```python
from build123d import *

# Parameters (mm, degrees)
F2_T = -2.54


with BuildPart() as f1:
    # F0 (on Right) → F1 (revolve)
    with BuildSketch(Plane.YZ):
        with BuildLine():
            Line((-101.6, 0), (0, 0))
            Line((0, 0), (0, 635))
            Line((0, 635), (-79.028264, 460.275492))
            ThreePointArc((-79.028264, 460.275492), (-95.892951, 409.140737), (-101.6, 355.6))
            Line((-101.6, 355.6), (-101.6, 0))
        make_face()
    revolve(axis=Axis((0, 0, 317.5), (0, 0, 1)))

    # F2
    f2_openings = [f1.faces().sort_by_distance(p)[0] for p in [
        (0, 0, 0),
    ]]
    offset(amount=F2_T, openings=f2_openings)


solid = f1.part
```
CAD build for the part. Positions are in the model's coordinates, mm. Round coordinates to 2 decimals unless told otherwise and drop trailing zeros. Write each loop counter-clockwise with the first axis right and the second up, starting at its lowest first coordinate (ties: lowest second). Pieces come first, ordered by that corner, then holes. Notation, with made-up numbers: (80, 42) -> (99, 42) arc R20 cw to (99, 63) -> close; hole circle Ø8 at (-6, -30.75). An arc over 180 degrees is marked (long way). Answer in a Markdown table with one row per item. Add a question column.
Item 1: Mould opens along Y. For faces 1 (the face through (-99.184, 22.025, 175.311)), 2 (the face through (30.1, 4, 561.7)), 3 (the face through (98.217, 12.896, 175.311)), 4 (the face through (-97, -22, 0)) say: pulls with the +Y half, pulls with the -Y half, needs draft (parallel to the pull), parting line crosses it, or undercut.
Item 2: Saw through at A-A, the plane z = 195. Write the cut outline in (x, y).
Item 3: Drill centre lines: line 1 (X direction, y = 0, z = 227); line 2 (X direction, y = 20.5, z = 464); line 3 (Y direction, x = 44.5, z = 170). Where is each one in solid material? Low to high. Write a range as from..to.
Item 4: Drop flat-ended pins along their axis: pin 1 Ø1 at (x, z) = (-67.5, 178) entering from +Y; pin 2 Ø12 at (x, z) = (77, 123.5) entering from -Y; pin 3 Ø4 at (x, z) = (-2.5, 534.5) entering from +Y. Give the stop position or say it passes through.
Findings below:
| question | item | result |
|---|---|---|
| 1 | face 1 | parting line crosses it |
| 1 | face 2 | undercut |
| 1 | face 3 | undercut |
| 1 | face 4 | needs draft |
| 2 | outline | circle Ø203.2 at (0, 0); hole circle Ø198.12 at (0, 0) |
| 3 | line 1 | x = -101.6..-99.06, 99.06..101.6 |
| 3 | line 2 | x = -74.58..-71.68, 71.68..74.58 |
| 3 | line 3 | y = -91.34..-88.5, 88.5..91.34 |
| 4 | pin 1 | stops at y = 76.38 |
| 4 | pin 2 | stops at y = -72.67 |
| 4 | pin 3 | stops at y = 46.3 |
